Can you work these out from the model? Positions are in its coordinate system, mm. Face numbers are marked on the shaded views. A direction names the side the tool comes from. Coordinates: 2 decimals unless noted, no trailing zeros. Loops run counter-clockwise (first coordinate to the right, second up) from the corner with the lowest first, then second, coordinate; pieces in that order, holes last. Notation, with made-up numbers: (71.25, -1) -> (78.25, -1) arc R21 ccw to (78.25, 16) -> close; hole circle Ø10 at (65.25, 1.25). An arc over 180 degrees is marked (long way). Use one line per item in the form item = value. Start each with the question number.
(1) Imagine slicing it at D-D (x = 31). List the corners of the cut face in (y, z) for me, plus the area to 3 significant figures.
(2) Imagine slicing it at C-C (z = 8.5). List the corners of the cut face in (x, y) for me, plus the area to 3 significant figures.
(3) I'm going to push a flat-ended pin straight in: pin 1 (3 mm diameter, centred on x = 32, z = 5, fed in from +Y). Where does the tip first touch, or does it pass through?
(4) I need wall thicknesses on line 1 (Y direction, x = 10, z = 2); line 2 (Z direction, x = 32, y = -38). Which ranges of each line are inside material? Lowest first, please. Write a range as [from, to].
(5) On a 3-axis mill with a long thin cutter (end or side, diameter ignored), from which of +Z, -Z, +X, -X, +Y, -Y can I reach the whole of each face in a straight line? I mean the marked faces 5 and 6. Say none if no direction works.
(6) Thinking about a two-plate mould opening in Z: for the marked faces 1, 2, 3 and 4, which applies, released by +Z, released by -Z, zero draft, split by the parting line, or undercut?
(7) Imagine slicing it at A-A (y = -12). List the corners of the cut face in (x, z) for me.
(8) Imagine slicing it at B-B (x = 10). List the corners of the cut face in (y, z) for me, plus the area to 3 significant figures.
Autodesk Inventor part; units mm, degrees
ref_plane "YZ Plane" through (0, 0, 0) normal (1, 0, 0) x (0, 1, 0)
ref_plane "XZ Plane" through (0, 0, 0) normal (0, 1, 0) x (-1, 0, 0)
ref_plane "XY Plane" through (0, 0, 0) normal (0, 0, 1) x (1, 0, 0)
sketch "草图1" plane through (0, 0, 0) normal (0, 0, 1) x (1, 0, 0)
  line L0 (0, 0) -> (27, 0)
  line L1 (27, 0) -> (27, -45)
  line L2 (27, -45) -> (0, -45)
  line L3 (0, -45) -> (0, 0)
  dimension "d0" = 27
  dimension "d1" = 45
extrude "拉伸1" add sketch "草图1" along normal blind 10
sketch "草图2" plane through (0, 0, 0) normal (0, 1, 0) x (1, 0, 0)
  circle A0 centre (32, -5) radius 5
  line L0 (27, -10) -> (0, -10)
  line L1 (27, 0) -> (27, -10)
  line L2 (0, 0) -> (27, 0)
  line L3 (32, 0) -> (27, 0)
  line L4 (27, 0) -> (27, -10)
  line L5 (27, -5) -> (27, 0)
  dimension "d4" = 10
  dimension "d5" = 5
  dimension "d6" = 5
extrude "拉伸2" add sketch "草图2" against normal blind 15
sketch "草图3" plane through (0, 0, 10) normal (0, 1, 0) x (1, 0, 0)
  arc A0 (27, 5) -> (32, 10) centre (32, 5) ccw
  circle A1 centre (32, 5) radius 2.5
  point P0 (0, 10)
  dimension "d9" = 5
ref_plane "工作平面1" through (0, -22.5, 0) normal (0, -1, 0) x (1, 0, 0)
mirror "镜像1" about plane through (0, -22.5, 0) normal (0, -1, 0) of "拉伸2"
extrude "拉伸3" cut sketch "草图3" against normal up to surface (45 mm away)
sketch "草图4" plane through (0, 0, 10) normal (0, 0, 1) x (1, 0, 0)
  line L0 (27, 0) -> (0, 0)
  line L1 (0, -45) -> (27, -45)
  line L2 (0, 0) -> (0, -45)
  point P0 (10, -12)
  point P1 (10, -33)
  dimension "d12" = 12
  dimension "d13" = 12
  dimension "d14" = 10
  dimension "d15" = 10
hole "孔1" at (10, -12, 10) at (10, -33, 10) direction (0, 0, -1) diameter 8.376 depth 27.3
properties part number "连接块"
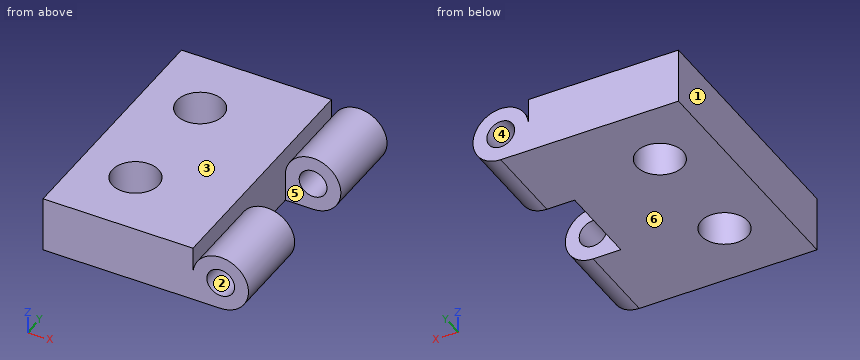
Worked out:
q1.outline = (-45, 0) -> (-30, 0) -> (-30, 2.71) -> (-45, 2.71) -> close; (-45, 7.29) -> (-30, 7.29) -> (-30, 9.9) -> (-45, 9.9) -> close; (-15, 0) -> (0, 0) -> (0, 2.71) -> (-15, 2.71) -> close; (-15, 7.29) -> (0, 7.29) -> (0, 9.9) -> (-15, 9.9) -> close
q1.area = 159 mm2
q2.outline = (0, -45) -> (27, -45) -> (27, 0) -> (0, 0) -> close; (28.43, -45) -> (35.57, -45) -> (35.57, -30) -> (28.43, -30) -> close; (28.43, -15) -> (35.57, -15) -> (35.57, 0) -> (28.43, 0) -> close; hole circle Ø8.38 at (10, -33); hole circle Ø8.38 at (10, -12)
q2.area = 1,320 mm2
q3.pin_1 = through
q4.line_1 = [-45, -37.19], [-28.81, -16.19], [-7.81, 0]
q4.line_2 = [0, 2.5], [7.5, 10]
q5.face_5 = +Z, -Z, +X
q5.face_6 = -Z, +X, -X, +Y, -Y
q6.face_1 = zero draft
q6.face_2 = undercut
q6.face_3 = released by +Z
q6.face_4 = undercut
q7.outline = (0, 0) -> (5.81, 0) -> (5.81, 10) -> (0, 10) -> close; (14.19, 0) -> (32, 0) arc R5 ccw (long way) to (27, 5) -> (27, 10) -> (14.19, 10) -> close; hole circle Ø5 at (32, 5)
q8.outline = (-45, 0) -> (-37.19, 0) -> (-37.19, 10) -> (-45, 10) -> close; (-28.81, 0) -> (-16.19, 0) -> (-16.19, 10) -> (-28.81, 10) -> close; (-7.81, 0) -> (0, 0) -> (0, 10) -> (-7.81, 10) -> close
q8.area = 282 mm2
